Part model, mm, in its own coordinate system. Face numbers are marked on the shaded views. A direction names the side the tool comes from. Coordinates: 2 decimals unless noted, no trailing zeros. Loops run counter-clockwise (first coordinate to the right, second up) from the corner with the lowest first, then second, coordinate; pieces in that order, holes last. Notation, with made-up numbers: M -5,-22.5 L 14,-22.5 A29 ccw 14,16.5 Z; hole C 74.25,30.25 d2. An arc over 180 degrees is marked long. Answer as CSV lines item,"result". Start each with the question number.
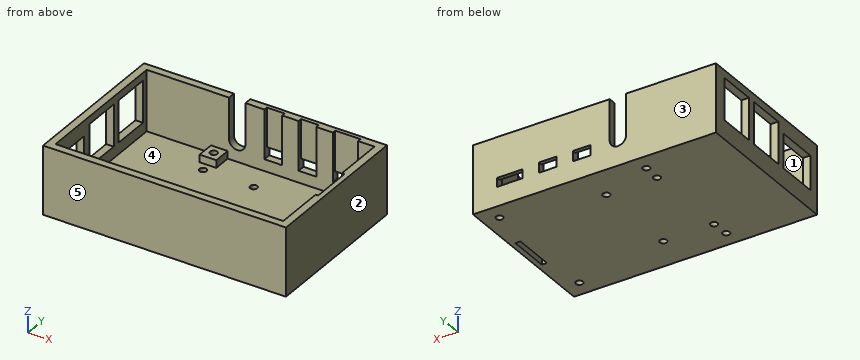
from build123d import *

# Parameters (mm, degrees)
SKETCH_1_W               = 90
SKETCH_1_H               = 56
SKETCH_1_R               = 1.4
EXTRUDE_1_DEPTH          = 3
SKETCH_2_W               = 6.6
SKETCH_2_H               = 7
SKETCH_2_R               = 1.4
EXTRUDE_2_DEPTH          = 3
SKETCH_3_W               = 96
SKETCH_3_H               = 62
SKETCH_3_W_2             = 90
SKETCH_3_H_2             = 56
EXTRUDE_3_DEPTH          = 27
SKETCH_4_W               = 16.5
SKETCH_4_H               = 15
SKETCH_4_W_2             = 13.5
SKETCH_4_H_2             = 16.5
CUT_EXTRUDE_1_DEPTH      = 3
CUT_EXTRUDE_2_REACH      = 84.928
SKETCH_5_W               = 10
SKETCH_5_H               = 3.5
SKETCH_5_W_2             = 7
SKETCH_5_H_2             = 4
CUT_EXTRUDE_3_REACH      = 65.198
SKETCH_6_W               = 7
SKETCH_6_H               = 1.5
SKETCH_6_W_2             = 10
CUT_EXTRUDE_6_DEPTH      = 64.198101237
CUT_EXTRUDE_6_DEPTH_BACK = 5
SKETCH_7_W               = 2
SKETCH_7_H               = 16.2
SKETCH_8_R               = 1.4
CUT_EXTRUDE_7_DEPTH      = 5


with BuildPart() as part:
    # 스케치1 → 보스-돌출1 (new body)
    with BuildSketch(Plane.XY):
        Rectangle(SKETCH_1_W, SKETCH_1_H)
        with Locations((-16.3, 24.5)):
            Circle(SKETCH_1_R, mode=Mode.SUBTRACT)
        with Locations((41.7, 24.5)):
            Circle(SKETCH_1_R, mode=Mode.SUBTRACT)
        with Locations(Location((41.7, -24.5, 0), (0, 0, 180))):
            Circle(SKETCH_1_R, mode=Mode.SUBTRACT)
        with Locations(Location((-16.3, -24.5, 0), (0, 0, 180))):
            Circle(SKETCH_1_R, mode=Mode.SUBTRACT)
    extrude(amount=EXTRUDE_1_DEPTH)

    # 스케치2 → 보스-돌출2 (add)
    # profile 1 of 4: a face of its own
    with BuildSketch(Plane.XY.offset(3)):
        with Locations((-16.3, 24.5)):
            Rectangle(SKETCH_2_W, SKETCH_2_H)
        with Locations((-16.3, 24.5)):
            Circle(SKETCH_2_R, mode=Mode.SUBTRACT)
    # profile 2 of 4: a face of its own
    with BuildSketch(Plane.XY.offset(3)):
        with Locations((41.7, 24.5)):
            Rectangle(SKETCH_2_W, SKETCH_2_H)
        with Locations((41.7, 24.5)):
            Circle(SKETCH_2_R, mode=Mode.SUBTRACT)
    # profile 3 of 4: a face of its own
    with BuildSketch(Plane.XY.offset(3)):
        with Locations((41.7, -24.5)):
            Rectangle(SKETCH_2_W, SKETCH_2_H)
        with Locations(Location((41.7, -24.5, 0), (0, 0, 180))):
            Circle(SKETCH_2_R, mode=Mode.SUBTRACT)
    # profile 4 of 4: a face of its own
    with BuildSketch(Plane.XY.offset(3)):
        with Locations((-16.3, -24.5)):
            Rectangle(SKETCH_2_W, SKETCH_2_H)
        with Locations(Location((-16.3, -24.5, 0), (0, 0, 180))):
            Circle(SKETCH_2_R, mode=Mode.SUBTRACT)
    extrude(amount=EXTRUDE_2_DEPTH)

    # 스케치3 → 보스-돌출3 (add)
    with BuildSketch(Plane.XY):
        Rectangle(SKETCH_3_W, SKETCH_3_H)
        Rectangle(SKETCH_3_W_2, SKETCH_3_H_2, mode=Mode.SUBTRACT)
    extrude(amount=EXTRUDE_3_DEPTH)

    # 스케치4 → 컷-돌출1 (cut)
    with BuildSketch(Plane.ZY.offset(48)):
        with Locations((15.75, 18.280682484)):
            Rectangle(SKETCH_4_W, SKETCH_4_H)
        with Locations((15.75, 0.280682484)):
            Rectangle(SKETCH_4_W, SKETCH_4_H)
        with Locations((14.25, -18.669317516)):
            Rectangle(SKETCH_4_W_2, SKETCH_4_H_2)
    extrude(amount=-CUT_EXTRUDE_1_DEPTH, mode=Mode.SUBTRACT)

    # 스케치5 → 컷-돌출2 (cut, up to next)
    with BuildSketch(Plane(origin=(0, 31, 0), x_dir=(1, 0, 0), z_dir=(0, 1, 0)), mode=Mode.PRIVATE) as cut_extrude_2_sk1:
        with Locations((33.5, -9.35)):
            Rectangle(SKETCH_5_W, SKETCH_5_H)
    cut_extrude_2_tool1 = extrude(cut_extrude_2_sk1.sketch, amount=-CUT_EXTRUDE_2_REACH, mode=Mode.PRIVATE) & part.part
    # 스케치5 → 컷-돌출2 (cut, up to next)
    with BuildSketch(Plane(origin=(0, 31, 0), x_dir=(1, 0, 0), z_dir=(0, 1, 0)), mode=Mode.PRIVATE) as cut_extrude_2_sk2:
        with Locations((18.5, -9.6)):
            Rectangle(SKETCH_5_W_2, SKETCH_5_H_2)
    cut_extrude_2_tool2 = extrude(cut_extrude_2_sk2.sketch, amount=-CUT_EXTRUDE_2_REACH, mode=Mode.PRIVATE) & part.part
    # 스케치5 → 컷-돌출2 (cut, up to next)
    with BuildSketch(Plane(origin=(0, 31, 0), x_dir=(1, 0, 0), z_dir=(0, 1, 0)), mode=Mode.PRIVATE) as cut_extrude_2_sk3:
        with Locations((5, -9.6)):
            Rectangle(SKETCH_5_W_2, SKETCH_5_H_2)
    cut_extrude_2_tool3 = extrude(cut_extrude_2_sk3.sketch, amount=-CUT_EXTRUDE_2_REACH, mode=Mode.PRIVATE) & part.part
    # 스케치5 → 컷-돌출2 (cut, up to next)
    with BuildSketch(Plane(origin=(0, 31, 0), x_dir=(1, 0, 0), z_dir=(0, 1, 0)), mode=Mode.PRIVATE) as cut_extrude_2_sk4:
        with BuildLine():
            Line((-12.5, -10.85), (-12.5, -27))
            Line((-12.5, -27), (-6, -27))
            Line((-6, -27), (-6, -10.85))
            ThreePointArc((-6, -10.85), (-9.25, -7.6), (-12.5, -10.85))
        make_face()
    cut_extrude_2_tool4 = extrude(cut_extrude_2_sk4.sketch, amount=-CUT_EXTRUDE_2_REACH, mode=Mode.PRIVATE) & part.part
    add(cut_extrude_2_tool1.solids().sort_by_distance((33.5, 31, 9.35))[0], mode=Mode.SUBTRACT)
    add(cut_extrude_2_tool2.solids().sort_by_distance((18.5, 31, 9.6))[0], mode=Mode.SUBTRACT)
    add(cut_extrude_2_tool3.solids().sort_by_distance((5, 31, 9.6))[0], mode=Mode.SUBTRACT)
    add(cut_extrude_2_tool4.solids().sort_by_distance((-9.25, 31, 17.634661))[0], mode=Mode.SUBTRACT)

    # 스케치6 → 컷-돌출3 (cut, up to next)
    with BuildSketch(Plane.XY.offset(27), mode=Mode.PRIVATE) as cut_extrude_3_sk1:
        with Locations((5, 28.75)):
            Rectangle(SKETCH_6_W, SKETCH_6_H)
    cut_extrude_3_tool1 = extrude(cut_extrude_3_sk1.sketch, amount=-CUT_EXTRUDE_3_REACH, mode=Mode.PRIVATE) & part.part
    # 스케치6 → 컷-돌출3 (cut, up to next)
    with BuildSketch(Plane.XY.offset(27), mode=Mode.PRIVATE) as cut_extrude_3_sk2:
        with Locations((18.5, 28.75)):
            Rectangle(SKETCH_6_W, SKETCH_6_H)
    cut_extrude_3_tool2 = extrude(cut_extrude_3_sk2.sketch, amount=-CUT_EXTRUDE_3_REACH, mode=Mode.PRIVATE) & part.part
    # 스케치6 → 컷-돌출3 (cut, up to next)
    with BuildSketch(Plane.XY.offset(27), mode=Mode.PRIVATE) as cut_extrude_3_sk3:
        with Locations((33.5, 28.75)):
            Rectangle(SKETCH_6_W_2, SKETCH_6_H)
    cut_extrude_3_tool3 = extrude(cut_extrude_3_sk3.sketch, amount=-CUT_EXTRUDE_3_REACH, mode=Mode.PRIVATE) & part.part
    add(cut_extrude_3_tool1.solids().sort_by_distance((5, 28.75, 27))[0], mode=Mode.SUBTRACT)
    add(cut_extrude_3_tool2.solids().sort_by_distance((18.5, 28.75, 27))[0], mode=Mode.SUBTRACT)
    add(cut_extrude_3_tool3.solids().sort_by_distance((33.5, 28.75, 27))[0], mode=Mode.SUBTRACT)

    # 스케치7 → 컷-돌출6 (cut, two sides: drawn at the far end of the back side and taken through both)
    with BuildSketch(Plane.XY.offset(-CUT_EXTRUDE_6_DEPTH_BACK)):
        with Locations((45, 0)):
            Rectangle(SKETCH_7_W, SKETCH_7_H)
    extrude(amount=CUT_EXTRUDE_6_DEPTH + CUT_EXTRUDE_6_DEPTH_BACK, mode=Mode.SUBTRACT)

    # 스케치8 → 컷-돌출7 (cut)
    with BuildSketch(Plane(origin=(0, 0, 0), x_dir=(-1, 0, 0), z_dir=(0, 0, -1))):
        with Locations((-4, 17.5)):
            Circle(SKETCH_8_R)
        with Locations((16, 17.5)):
            Circle(SKETCH_8_R)
        with Locations(Location((-4, -17.5, 0), (0, 0, 180))):
            Circle(SKETCH_8_R)
        with Locations(Location((16, -17.5, 0), (0, 0, 180))):
            Circle(SKETCH_8_R)
    extrude(amount=-CUT_EXTRUDE_7_DEPTH, mode=Mode.SUBTRACT)


solid = part.part
Q1. Slice it at D-D, the plane x = 4. Write the cut outline in (y, z), and give its area (3 significant figures).
Q2. Wall check: L1, parallel to X at y = -24.5, z = 1.9; L2, parallel to Y at x = 18, z = 19.5; L3, parallel to Y at x = -3, z = 22.5. Give the ranges that are in metal, low to high.
Q3. Slice it at A-A, the plane y = -24.5. Write the cut outline in (x, z).
Q4. Flat gauge pins, fed straight in: P1, Ø0.8, axis at x = 32.5, y = 30.5, coming from the -Z side; P2, Ø17, axis at x = 9.5, y = 13, coming from the +Z side; P3, Ø5, axis at y = 0.5, z = 20, coming from the -X side; P4, Ø3.5, axis at x = 40.5, y = 23.5, coming from the +Z side. Where does each tip first touch, or does it go through?
Q5. Two-plate mould, pull along Y, no slides. Class the marked faces 3, 4 and 5: +Y half, -Y half, draft (parallel to the pull), parting line (faces both ways), or undercut.
Q6. Slice it at C-C, the plane y = 15. Write the cut outline in (x, z), and give its area (4 significant figures).
Q7. Slice it at B-B, the plane x = 34. Write the cut outline in (y, z), and give its area (3 significant figures).
Q8. Tool access for the marked faces 1 and 2: list every direction of +Z, -Z, +X, -X, +Y, -Y with a clear straight run to the whole face (end or side of a thin tool).
Solved:
1,outline,"M -31,0 L -18.9,0 L -18.9,3 L -28,3 L -28,27 L -31,27 Z; M -16.1,0 L 16.1,0 L 16.1,3 L -16.1,3 Z; M 18.9,0 L 31,0 L 31,7.6 L 28,7.6 L 28,3 L 18.9,3 Z; M 29.5,11.6 L 31,11.6 L 31,27 L 29.5,27 Z"
1,area,"278 mm2"
2,L1,"x = -48 to -17.7, -14.9 to 40.3, 43.1 to 48"
2,L2,"y = -31 to -28, 29.5 to 31"
2,L3,"y = -31 to -28, 28 to 31"
3,outline,"M -48,0 L -17.7,0 L -17.7,6 L -19.6,6 L -19.6,3 L -45,3 L -45,7.5 L -48,7.5 Z; M -48,21 L -45,21 L -45,27 L -48,27 Z; M -14.9,0 L 40.3,0 L 40.3,6 L 38.4,6 L 38.4,3 L -13,3 L -13,6 L -14.9,6 Z; M 43.1,0 L 48,0 L 48,27 L 45,27 L 45,6 L 43.1,6 Z"
4,P1,"stops at z = 0"
4,P2,"stops at z = 3"
4,P3,"stops at x = 46"
4,P4,"stops at z = 6"
5,face 3,"+Y half"
5,face 4,"undercut"
5,face 5,"-Y half"
6,outline,"M -48,0 L 48,0 L 48,27 L 45,27 L 45,3 L -45,3 L -45,7.5 L -48,7.5 Z; M -48,24 L -45,24 L -45,27 L -48,27 Z"
6,area,"382.5 mm2"
7,outline,"M -31,0 L 31,0 L 31,7.6 L 28,7.6 L 28,3 L -28,3 L -28,27 L -31,27 Z; M 29.5,11.1 L 31,11.1 L 31,27 L 29.5,27 Z"
7,area,"296 mm2"
8,face 1,"+Z"
8,face 2,"+Z, -Z, +X, +Y, -Y"
